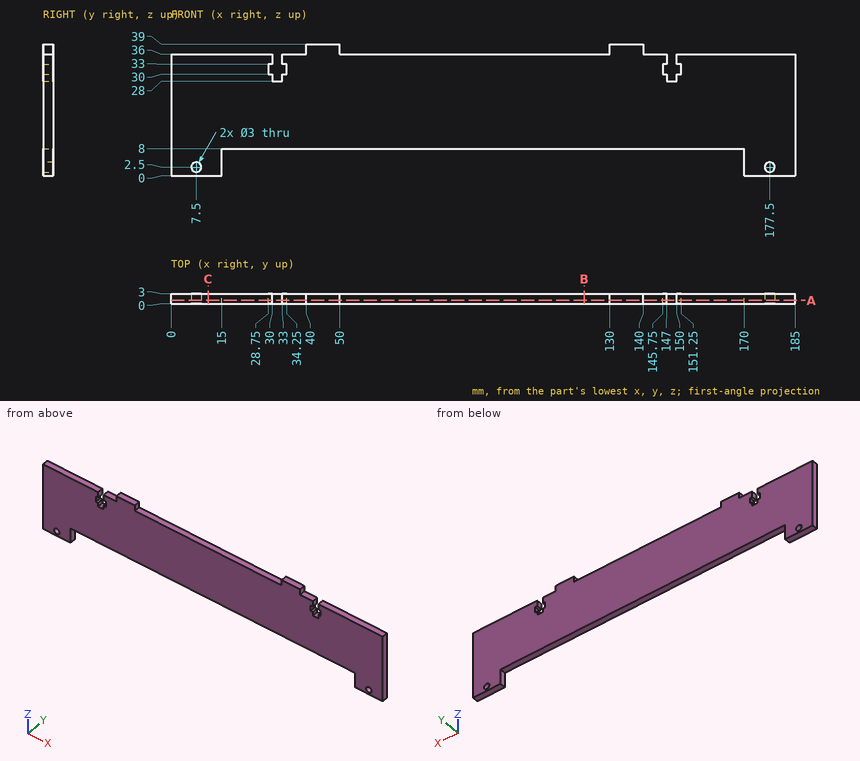
Drawing for the job (mm, zero at the part's lowest x, y, z). Round coordinates to 2 decimals unless told otherwise and drop trailing zeros. Loops run counter-clockwise (first coordinate to the right, second up) from the corner with the lowest first, then second, coordinate; pieces in that order, holes last. Notation, with made-up numbers: M 46.25,76 L 94.25,76 A20 cw 94.25,99 Z; hole C 82,-12.5 d4. An arc over 180 degrees is marked long. Use a Markdown table: item, result. Add a question column.
(1) Drill centre lines: line 1 (X direction, y = 2.5, z = 34.5); line 2 (X direction, y = 1.95, z = 2.5); line 3 (X direction, y = 1.45, z = 31). Where is each one in solid material? Low to high.
(2) Cut at C-C (x = 11). Give the cut face in (y, z).
(3) Flat gauge pins, fed straight in: pin 1 (0.9 mm diameter, centred on x = 75, y = 2, fed in from +Z); pin 2 (0.6 mm diameter, centred on x = 146.5, y = 2, fed in from -Z). Where does each tip first touch, or does it go through?
(4) Cut at A-A (y = 1). State how many separate pieces and enclosed holes the cut face has, and give its area (3 significant figures).
(5) Cut at B-B (x = 122.5). Give the cut face in (y, z).
Geometry says:
| question | item | result |
|---|---|---|
| 1 | line 1 | x = 0 to 30, 33 to 147, 150 to 185 |
| 1 | line 2 | x = 0 to 6, 9 to 15, 170 to 176, 179 to 185 |
| 1 | line 3 | x = 0 to 28.75, 34.25 to 145.75, 151.25 to 185 |
| 2 | outline | M 0,0 L 3,0 L 3,36 L 0,36 Z |
| 3 | pin 1 | stops at z = 36 |
| 3 | pin 2 | stops at z = 8 |
| 4 | separate pieces | 1 |
| 4 | enclosed holes | 2 |
| 4 | area | 5,400 mm² |
| 5 | outline | M 0,8 L 3,8 L 3,36 L 0,36 Z |
